```python
from build123d import *

# Parameters (mm, degrees)
SKETCH1_R          = 4.7625
SKETCH1_R_2        = 3.175
EXTRUDE1_DEPTH     = 15.24
SKETCH2_R          = 3.175
EXTRUDE2_DEPTH     = 3.175
SKETCH3_R          = 4.7625
SKETCH3_R_2        = 3.175
EXTRUDE3_DEPTH     = 31.75
SKETCH4_R          = 7.366
SKETCH4_R_2        = 5.588
CUT_EXTRUDE1_DEPTH = 1.5875
SKETCH5_R          = 5.588
SKETCH5_R_2        = 4.7625
EXTRUDE4_DEPTH     = 6.35
SKETCH8_R          = 5.588
SKETCH8_R_2        = 4.7625
EXTRUDE5_DEPTH     = 6.35
SKETCH9_R          = 5.588
SKETCH9_R_2        = 4.7625
EXTRUDE6_DEPTH     = 12.7


with BuildPart() as part:
    # Sketch1 → Extrude1 (new body)
    with BuildSketch(Plane(origin=(0, 0, 0), x_dir=(1, 0, 0), z_dir=(0, 1, 0))):
        Circle(SKETCH1_R)
        Circle(SKETCH1_R_2, mode=Mode.SUBTRACT)
    extrude(amount=EXTRUDE1_DEPTH)

    # Sketch2 → Extrude2 (add)
    with BuildSketch(Plane.XZ):
        Polygon((9.525, 5.499261314), (9.525, -5.499261314), (0, -10.998522628), (-9.525, -5.499261314), (-9.525, 5.499261314), (0, 10.998522628), align=None)
        Circle(SKETCH2_R, mode=Mode.SUBTRACT)
    extrude(amount=EXTRUDE2_DEPTH)

    # Sketch3 → Extrude3 (add)
    with BuildSketch(Plane.XZ.offset(3.175)):
        Circle(SKETCH3_R)
        Circle(SKETCH3_R_2, mode=Mode.SUBTRACT)
    extrude(amount=EXTRUDE3_DEPTH)

    # Sketch4 → Cut-Extrude1 (cut)
    with BuildSketch(Plane.XZ.offset(3.175)):
        Circle(SKETCH4_R)
        Circle(SKETCH4_R_2, mode=Mode.SUBTRACT)
    extrude(amount=-CUT_EXTRUDE1_DEPTH, mode=Mode.SUBTRACT)

    # Sketch5 → Extrude4 (add)
    with BuildSketch(Plane(origin=(0, 15.24, 0), x_dir=(-1, 0, 0), z_dir=(0, 1, 0))):
        Circle(SKETCH5_R)
        Circle(SKETCH5_R_2, mode=Mode.SUBTRACT)
    extrude(amount=-EXTRUDE4_DEPTH)

    # Sketch8 → Extrude5 (add)
    with BuildSketch(Plane.XZ.offset(34.925)):
        Circle(SKETCH8_R)
        Circle(SKETCH8_R_2, mode=Mode.SUBTRACT)
    extrude(amount=-EXTRUDE5_DEPTH)

    # Sketch7 → Cut-Revolve1 (revolve, cut)
    with BuildSketch(Plane(origin=(0, 0, 0), x_dir=(0, 0, -1), z_dir=(1, 0, 0))):
        Polygon((-5.588, 8.89), (-4.7625, 15.24), (-5.588, 15.24), align=None)
        Polygon((-5.588, -34.925), (-5.588, -28.575), (-4.7625, -34.925), align=None)
    revolve(axis=Axis((0, 15.24, 0), (0, -1, 0)), mode=Mode.SUBTRACT)

    # Sketch9 → Extrude6 (add)
    with BuildSketch(Plane.XZ.offset(3.175)):
        Circle(SKETCH9_R)
        Circle(SKETCH9_R_2, mode=Mode.SUBTRACT)
    extrude(amount=EXTRUDE6_DEPTH)


solid = part.part
```
Verification items for the finished model (mm, model axes). A direction names the side the tool comes from. Give positions to 0.01 mm unless a question says otherwise; leave off trailing zeros. Order: outer loops, then holes, each group sorted by start corner. A loop starts at its lowest first (then second) coordinate and runs counter-clockwise, first axis right, second up. Notation, with made-up numbers: M 34,-10 L 53,-10 A26 ccw 53,11 Z; hole C 64,-6 d7. An arc over 180 degrees is marked long. Answer in a Markdown table with one row per item. Add a question column.
Item 1: Gauge pin test, flat ends, axial feed: pin 1 (2 mm diameter, centred on y = -28, z = 8.5, fed in from +X); pin 2 (10 mm diameter, centred on x = 3.5, y = 8, fed in from +Z); pin 3 (2 mm diameter, centred on x = 4, y = 0, fed in from -Z). Record the tip position at first contact, or that the pin passes through.
Item 2: Mould release check, pull along Y, two halves, no side actions. Record for faces 1 (the conical face through (-5.035, -32.5, -0.661)), 2 (the flat face through (-4, 8.89, 3)), 3 (the flat face through (4.696, -1.565, 8.287)): released by +Y, released by -Y, zero draft, split by the parting line, or undercut.
Item 3: Section check B-B, the plane y = -4.5. Enter the section's corners in (x, z) (3 decimals).
Item 4: Tool access check on faces 4 (the flat face through (-3, -3.175, 7)), 5 (the flat face through (4, -28.575, 3)), 6 (the flat face through (9.525, -2, 0)). Record the directions out of +Z, -Z, +X, -X, +Y, -Y that give a thin tool (end or side, any length) a straight path to the whole face; none if there is none.
Item 5: Section check C-C, the plane x = -8. Enter the section's corners in (y, z) (3 decimals), and give its area (3 significant figures).
Item 6: Scan lines: probe 1 along Z at (x, y) = (0, -2.45) (3 decimals); probe 2 along X at (y, z) = (2, 0) (1 decimal); probe 3 along Z at (x, y) = (0, -11) (3 decimals). Record each from-to range of solid material in increasing order. Write a range as from..to.
Filled sheet:
| question | item | result |
|---|---|---|
| 1 | pin 1 | passes through |
| 1 | pin 2 | stops at z = 5.59 |
| 1 | pin 3 | stops at z = -9.27 |
| 2 | face 1 | released by -Y |
| 2 | face 2 | undercut |
| 2 | face 3 | zero draft |
| 3 | outline | C 0,0 d11.176; hole C 0,0 d6.35 |
| 4 | face 4 | -Y |
| 4 | face 5 | none |
| 4 | face 6 | +Z, -Z, +X, +Y, -Y |
| 5 | outline | M -3.175,-6.38 L 0,-6.38 L 0,6.38 L -3.175,6.38 Z |
| 5 | area | 40.5 mm^2 |
| 6 | probe 1 | z = -10.999..-7.366, -5.588..-3.175, 3.175..5.588, 7.366..10.999 |
| 6 | probe 2 | x = -4.8..-3.2, 3.2..4.8 |
| 6 | probe 3 | z = -5.588..-3.175, 3.175..5.588 |
